from build123d import *

# Parameters (mm, degrees)
BOSS_EXTRU_2_DEPTH      = 30
COQUE2_T                = -2
ESQUISSE11_W            = 2
ESQUISSE11_H            = 30
ENL_V_MAT_EXTRU_2_DEPTH = 5
ESQUISSE17_W            = 15
ESQUISSE17_H            = 32
ENL_V_MAT_EXTRU_3_DEPTH = 10


with BuildPart() as part:
    # Esquisse5 → Boss.-Extru.2 (new, symmetric)
    with BuildSketch(Plane.XY):
        with BuildLine():
            Line((-50, -35), (50, -35))
            ThreePointArc((50, -35), (57.071067812, -32.071067812), (60, -25))
            Line((60, -25), (60, 25))
            ThreePointArc((60, 25), (57.071067812, 32.071067812), (50, 35))
            Line((50, 35), (-50, 35))
            ThreePointArc((-50, 35), (-57.071067812, 32.071067812), (-60, 25))
            Line((-60, 25), (-60, -25))
            ThreePointArc((-60, -25), (-57.071067812, -32.071067812), (-50, -35))
        make_face()
    extrude(amount=BOSS_EXTRU_2_DEPTH, both=True)

    # Coque2
    coque2_openings = [part.faces().sort_by_distance(p)[0] for p in [
        (0, 0, 30),
    ]]
    offset(amount=COQUE2_T, openings=coque2_openings, kind=Kind.INTERSECTION)

    # Enlèvement de matière-Balayage11: sweep along a path in Esquisse5<5>
    with BuildLine(Plane.XY) as enl_vement_de_mati_re_balayage11_path:
        Line((-50, -35), (50, -35))
        ThreePointArc((50, -35), (57.071067812, -32.071067812), (60, -25))
        Line((60, -25), (60, 25))
        ThreePointArc((60, 25), (57.071067812, 32.071067812), (50, 35))
        Line((50, 35), (-50, 35))
        ThreePointArc((-50, 35), (-57.071067812, 32.071067812), (-60, 25))
        Line((-60, 25), (-60, -25))
        ThreePointArc((-60, -25), (-57.071067812, -32.071067812), (-50, -35))
    # Esquisse11 → Enlèvement de matière-Balayage11 (sweep, cut)
    with BuildSketch(Plane(origin=(0, 0, 0), x_dir=(1, 0, 0), z_dir=(0, 1, 0))):
        with Locations((-60, 0)):
            Rectangle(ESQUISSE11_W, ESQUISSE11_H)
    sweep(path=enl_vement_de_mati_re_balayage11_path.line, mode=Mode.SUBTRACT)

    # Esquisse16 → Enlèv. mat.-Extru.2 (cut, symmetric)
    with BuildSketch(Plane.XZ.offset(34)):
        with BuildLine():
            Line((22.996916051, 12), (44.996916051, 12))
            ThreePointArc((44.996916051, 12), (46.996916051, 10), (44.996916051, 8))
            Line((44.996916051, 8), (22.996916051, 8))
            ThreePointArc((22.996916051, 8), (20.996916051, 10), (22.996916051, 12))
        make_face()
        with BuildLine():
            Line((-11.003083949, 12), (10.996916051, 12))
            ThreePointArc((10.996916051, 12), (12.996916051, 10), (10.996916051, 8))
            Line((10.996916051, 8), (-11.003083949, 8))
            ThreePointArc((-11.003083949, 8), (-13.003083949, 10), (-11.003083949, 12))
        make_face()
        with BuildLine():
            Line((-45, 12), (-23, 12))
            ThreePointArc((-23, 12), (-21, 10), (-23, 8))
            Line((-23, 8), (-45, 8))
            ThreePointArc((-45, 8), (-47, 10), (-45, 12))
        make_face()
        with BuildLine():
            Line((22.996916051, 0), (44.996916051, 0))
            ThreePointArc((44.996916051, 0), (46.996916051, 2), (44.996916051, 4))
            Line((44.996916051, 4), (22.996916051, 4))
            ThreePointArc((22.996916051, 4), (20.996916051, 2), (22.996916051, 0))
        make_face()
        with BuildLine():
            Line((-11.003083949, 0), (10.996916051, 0))
            ThreePointArc((10.996916051, 0), (12.996916051, 2), (10.996916051, 4))
            Line((10.996916051, 4), (-11.003083949, 4))
            ThreePointArc((-11.003083949, 4), (-13.003083949, 2), (-11.003083949, 0))
        make_face()
        with BuildLine():
            Line((-45, 0), (-23, 0))
            ThreePointArc((-23, 0), (-21, 2), (-23, 4))
            Line((-23, 4), (-45, 4))
            ThreePointArc((-45, 4), (-47, 2), (-45, 0))
        make_face()
        with BuildLine():
            Line((-45, -8), (-23, -8))
            ThreePointArc((-23, -8), (-21, -10), (-23, -12))
            Line((-23, -12), (-45, -12))
            ThreePointArc((-45, -12), (-47, -10), (-45, -8))
        make_face()
        with BuildLine():
            Line((-11.003083949, -8), (10.996916051, -8))
            ThreePointArc((10.996916051, -8), (12.996916051, -10), (10.996916051, -12))
            Line((10.996916051, -12), (-11.003083949, -12))
            ThreePointArc((-11.003083949, -12), (-13.003083949, -10), (-11.003083949, -8))
        make_face()
        with BuildLine():
            Line((22.996916051, -8), (44.996916051, -8))
            ThreePointArc((44.996916051, -8), (46.996916051, -10), (44.996916051, -12))
            Line((44.996916051, -12), (22.996916051, -12))
            ThreePointArc((22.996916051, -12), (20.996916051, -10), (22.996916051, -8))
        make_face()
    extrude(amount=ENL_V_MAT_EXTRU_2_DEPTH, both=True, mode=Mode.SUBTRACT)

    # Esquisse17 → Enlèv. mat.-Extru.3 (cut)
    with BuildSketch(Plane(origin=(60, 0, 0), x_dir=(0, 0, -1), z_dir=(1, 0, 0))):
        with Locations((18.5, 4)):
            Rectangle(ESQUISSE17_W, ESQUISSE17_H)
    extrude(amount=-ENL_V_MAT_EXTRU_3_DEPTH, mode=Mode.SUBTRACT)


solid = part.part
Work out the finished part from the listing and answer in its coordinate system (mm). A direction names the side the tool comes from. Round coordinates to 2 decimals unless told otherwise and drop trailing zeros. Write each loop counter-clockwise with the first axis right and the second up, starting at its lowest first coordinate (ties: lowest second). Pieces come first, ordered by that corner, then holes. Notation, with made-up numbers: (48, 83) - (72, 83) arc R35 ccw to (72, 120) - close; hole circle Ø5 at (13, 53). An arc over 180 degrees is marked (long way). Answer in a Markdown table with one row per item. Add a question column.
1. For faces 4 (the flat face through (59, 0, 0)), 5 (the cylindrical face through (55.594, -30.719, 1.406)), 6 (the cylindrical face through (-56.434, -31.294, -0.21)), 7 (the cylindrical face through (56.434, 31.294, -0.21)), determine the directions among +Z, -Z, +X, -X, +Y, -Y from which every point of the face is accessible in a straight line to the end or side of a thin tool.
2. A cutting plane is placed at A-A, the plane x = 2.5. Determine the outline of the cut face in (y, z).
3. A cutting plane is placed at C-C, the plane z = -20.5. Determine the outline of the cut face in (x, y).
4. A cutting plane is placed at D-D, the plane y = -22. Determine the outline of the cut face in (x, z), and give its area (3 significant figures).
5. Given pin 1 (1.6 mm diameter, centred on x = 59.5, z = -22, fed in from -Y); pin 2 (15 mm diameter, centred on y = 4.5, z = -11.5, fed in from +X); pin 3 (1.5 mm diameter, centred on y = -13, z = -2.5, fed in from -X); pin 4 (15 mm diameter, centred on y = 9, z = -9.5, fed in from -X), each flat-ended and moving along its own axis, determine where each tip first touches the part or whether it passes through.
6. Find the intervals of material crossed by line 1 along X through (y, z) = (-11, -6); line 2 along X through (y, z) = (3.5, 21.5); line 3 along Y through (x, z) = (-48, 13.5), in increasing order. Write a range as from..to.
7. A cutting plane is placed at B-B, the plane z = 10. Determine the outline of the cut face in (x, y), and give its area (3 significant figures).
8. The mould has two halves that part along X. Classify faces 1 (the flat face through (-60, 0, -22)), 2 (the cylindrical face through (56.294, -31.434, -0.21)), 3 (the cylindrical face through (-55.594, 30.719, 1.406)): +X half, -X half, draft (parallel to the pull), parting line (faces both ways), or undercut.
Worked out:
| question | item | result |
|---|---|---|
| 1 | face 4 | +X, +Y, -Y |
| 1 | face 5 | +Z |
| 1 | face 6 | -X, -Y |
| 1 | face 7 | +X, +Y |
| 2 | outline | (-35, -30) - (35, -30) - (35, -15) - (34, -15) - (34, 15) - (35, 15) - (35, 30) - (33, 30) - (33, -28) - (-33, -28) - (-33, -12) - (-34, -12) - (-34, -15) - (-35, -15) - close; (-35, 15) - (-34, 15) - (-34, 12) - (-33, 12) - (-33, 30) - (-35, 30) - close; (-34, -8) - (-33, -8) - (-33, 0) - (-34, 0) - close; (-34, 4) - (-33, 4) - (-33, 8) - (-34, 8) - close |
| 3 | outline | (-60, -25) arc R10 ccw to (-50, -35) - (50, -35) arc R10 ccw to (60, -25) - (60, -12) - (58, -12) - (58, -25) arc R8 cw to (50, -33) - (-50, -33) arc R8 cw to (-58, -25) - (-58, 25) arc R8 cw to (-50, 33) - (50, 33) arc R8 cw to (58, 25) - (58, 20) - (60, 20) - (60, 25) arc R10 ccw to (50, 35) - (-50, 35) arc R10 ccw to (-60, 25) - close |
| 4 | outline | (-60, -30) - (60, -30) - (60, -15) - (59, -15) - (59, 15) - (60, 15) - (60, 30) - (58, 30) - (58, -28) - (-58, -28) - (-58, 30) - (-60, 30) - (-60, 15) - (-59, 15) - (-59, -15) - (-60, -15) - close |
| 4 | area | 412 mm^2 |
| 5 | pin 1 | y = -29.93 |
| 5 | pin 2 | x = 59 |
| 5 | pin 3 | x = -59 |
| 5 | pin 4 | x = -60 |
| 6 | line 1 | -59..-58, 58..59 |
| 6 | line 2 | -60..-58, 58..60 |
| 6 | line 3 | -34..-33, 33..34 |
| 7 | outline | (-59, -25) arc R9 ccw to (-50, -34) - (-47, -34) - (-47, -33) - (-50, -33) arc R8 cw to (-58, -25) - (-58, 25) arc R8 cw to (-50, 33) - (50, 33) arc R8 cw to (58, 25) - (58, -25) arc R8 cw to (50, -33) - (47, -33) - (47, -34) - (50, -34) arc R9 ccw to (59, -25) - (59, 25) arc R9 ccw to (50, 34) - (-50, 34) arc R9 ccw to (-59, 25) - close; (-21, -34) - (-13, -34) - (-13, -33) - (-21, -33) - close; (13, -34) - (21, -34) - (21, -33) - (13, -33) - close |
| 7 | area | 275 mm^2 |
| 8 | face 1 | -X half |
| 8 | face 2 | +X half |
| 8 | face 3 | undercut |
